from build123d import *

# Parameters (mm, degrees)
SKETCH2_R           = 10.9
SKETCH2_R_2         = 1.55
BOSS_EXTRUDE1_DEPTH = 4.5
SKETCH3_R           = 6.25
SKETCH3_R_2         = 2.1
BOSS_EXTRUDE2_DEPTH = 6.5
CUT_EXTRUDE2_START  = -9.5
SKETCH6_R           = 2.1
CUT_EXTRUDE2_DEPTH  = 9.5
SKETCH7_R           = 3.6
CUT_EXTRUDE3_DEPTH  = 2.9
CUT_EXTRUDE4_DEPTH  = 2.8
CHAMFER2_SIZE       = 0.5
SKETCH11_R          = 1.55
CUT_EXTRUDE5_DEPTH  = 5.5
SKETCH14_W          = 2.8
SKETCH14_H          = 6.2
CUT_EXTRUDE6_DEPTH  = 6.4
CUT_EXTRUDE8_DEPTH  = 6.2
CHAMFER3_SIZE       = 0.4
CHAMFER4_SIZE       = 0.4
SKETCH19_W          = 2.5
SKETCH19_H          = 7
BOSS_EXTRUDE4_DEPTH = 10
FILLET5_R           = 3
CUT_EXTRUDE9_DEPTH  = 6.5
CUT_EXTRUDE10_START = -87
SKETCH21_R          = 1.55
CUT_EXTRUDE10_DEPTH = 87


with BuildPart() as part:
    # Sketch2 → Boss-Extrude1 (new body)
    with BuildSketch(Plane.XY):
        Circle(SKETCH2_R)
        with Locations((0, 8)):
            Circle(SKETCH2_R_2, mode=Mode.SUBTRACT)
        with Locations((0, -8)):
            Circle(SKETCH2_R_2, mode=Mode.SUBTRACT)
    extrude(amount=BOSS_EXTRUDE1_DEPTH)

    # Sketch3 → Boss-Extrude2 (add)
    with BuildSketch(Plane(origin=(0, 0, 0), x_dir=(-1, 0, 0), z_dir=(0, 0, -1))):
        with Locations(Location((0, 0, 0), (0, 0, 180))):
            Circle(SKETCH3_R)
        with Locations(Location((0, 0, 0), (0, 0, 180))):
            Circle(SKETCH3_R_2, mode=Mode.SUBTRACT)
    extrude(amount=BOSS_EXTRUDE2_DEPTH)

    # Sketch6 → Cut-Extrude2 (cut)
    with BuildSketch(Plane(origin=(0, 0, 0), x_dir=(-1, 0, 0), z_dir=(0, 0, -1)).offset(CUT_EXTRUDE2_START)):
        with Locations(Location((0, 0, 0), (0, 0, 180))):
            Circle(SKETCH6_R)
    extrude(amount=CUT_EXTRUDE2_DEPTH, mode=Mode.SUBTRACT)

    # Sketch7 → Cut-Extrude3 (cut)
    with BuildSketch(Plane.XY.offset(4.5)):
        Circle(SKETCH7_R)
    extrude(amount=-CUT_EXTRUDE3_DEPTH, mode=Mode.SUBTRACT)

    # Sketch8 → Cut-Extrude4 (cut)
    with BuildSketch(Plane.XY.offset(4.5)):
        Polygon((1.58395502, 5.181415279), (3.232943481, 7.962452926), (1.64898846, 10.781037646), (-1.58395502, 10.818584721), (-3.232943481, 8.037547074), (-1.64898846, 5.218962354), align=None)
        Polygon((3.233098906, -8.020119499), (1.633973451, -5.210113964), (-1.599125456, -5.189994464), (-3.233098906, -7.979880501), (-1.633973451, -10.789886036), (1.599125456, -10.810005536), align=None)
    extrude(amount=-CUT_EXTRUDE4_DEPTH, mode=Mode.SUBTRACT)

    # Chamfer2
    chamfer2_edges = [part.edges().sort_by_distance(p)[0] for p in [
        (-3.6, 0, 4.5),
    ]]
    chamfer(chamfer2_edges, length=CHAMFER2_SIZE)

    # Sketch11 → Cut-Extrude5 (cut, symmetric)
    with BuildSketch(Plane(origin=(-6.25, 0, 0), x_dir=(0, 1, 0), z_dir=(-1, 0, 0))):
        with Locations(Location((0, 3.215789821, 0), (0, 0, 270))):
            Circle(SKETCH11_R)
    extrude(amount=CUT_EXTRUDE5_DEPTH, both=True, mode=Mode.SUBTRACT)

    # Sketch14 → Cut-Extrude6 (cut)
    with BuildSketch(Plane(origin=(0, 0, -6.5), x_dir=(-1, 0, 0), z_dir=(0, 0, -1))):
        with Locations((3.35, 0)):
            Rectangle(SKETCH14_W, SKETCH14_H)
    extrude(amount=-CUT_EXTRUDE6_DEPTH, mode=Mode.SUBTRACT)

    # Sketch17 → Cut-Extrude8 (cut)
    with BuildSketch(Plane.XY.offset(1.7)):
        Polygon((1.655062081, 10.777427379), (-1.577791627, 10.822039496), (-3.232853707, 8.044612117), (-1.655062081, 5.222572621), (1.577791627, 5.177960504), (3.232853707, 7.955387883), align=None)
    extrude(amount=CUT_EXTRUDE8_DEPTH, mode=Mode.SUBTRACT)

    # Chamfer3
    chamfer3_edges = [part.edges().sort_by_distance(p)[0] for p in [
        (3.231903858, 7.96069959, 4.5),
        (-1.649987082, 5.220739361, 4.5),
        (1.581916776, 5.181438951, 4.5),
        (-3.231903858, 8.03930041, 4.5),
        (-3.231858971, 8.042832931, 4.5),
        (0.771107805, 5.189092426, 4.5),
        (2.049929575, 10.07116703, 4.5),
        (1.578835079, 5.179711564, 4.5),
        (3.231858971, 7.957167069, 4.5),
        (-2.81987127, 8.737654839, 4.5),
        (-2.048763464, 5.926747264, 4.5),
        (-1.653023892, 5.222544495, 4.5),
        (2.81987127, 7.262345161, 4.5),
        (-10.899984913, 0.01813521, 4.5),
        (8.259417425, -7.112807026, 4.5),
        (2.837704165, 8.665765509, 4.5),
        (-2.006564209, 10.105849554, 4.5),
        (-2.837704165, 7.334234491, 4.5),
        (-0.842282238, 5.20959335, 4.5),
        (1.995421926, 5.87535886, 4.5),
        (-2.437601998, -9.377738754, 4.5),
        (2.42507938, -9.399751703, 4.5),
        (2.433536179, -6.615116731, 4.5),
        (0.017423997, -5.200054214, 4.5),
        (-2.416112181, -6.584937483, 4.5),
    ]]
    chamfer(chamfer3_edges, length=CHAMFER3_SIZE)

    # Chamfer4
    chamfer4_edges = [part.edges().sort_by_distance(p)[0] for p in [
        (-2.1, 0, 1.6),
    ]]
    chamfer(chamfer4_edges, length=CHAMFER4_SIZE)

    # Sketch19 → Boss-Extrude4 (add)
    with BuildSketch(Plane(origin=(0, 0, -6.5), x_dir=(-1, 0, 0), z_dir=(0, 0, -1))):
        with Locations((6.327927724, 0)):
            Rectangle(SKETCH19_W, SKETCH19_H)
    extrude(amount=-BOSS_EXTRUDE4_DEPTH)

    # Fillet5
    fillet5_edges = [part.edges().sort_by_distance(p)[0] for p in [
        (-5.178078794, -3.5, -3.25),
        (-5.178078794, 3.5, -3.25),
    ]]
    fillet(fillet5_edges, radius=FILLET5_R)

    # Sketch20 → Cut-Extrude9 (cut)
    with BuildSketch(Plane(origin=(0, 0, -6.5), x_dir=(-1, 0, 0), z_dir=(0, 0, -1))):
        Polygon((1.674315781, 10.9), (-1.674315781, 10.9), (-3.348631561, 8), (-1.674315781, 5.1), (1.674315781, 5.1), (3.348631561, 8), align=None)
        Polygon((1.674315781, -5.1), (-1.674315781, -5.1), (-3.348631561, -8), (-1.674315781, -10.9), (1.674315781, -10.9), (3.348631561, -8), align=None)
    extrude(amount=-CUT_EXTRUDE9_DEPTH, mode=Mode.SUBTRACT)

    # Sketch21 → Cut-Extrude10 (cut)
    with BuildSketch(Plane(origin=(-5.077927724, 0, 0), x_dir=(0, 0, -1), z_dir=(1, 0, 0)).offset(CUT_EXTRUDE10_START)):
        with Locations(Location((3.215789821, 0, 0), (0, 0, 180))):
            Circle(SKETCH21_R)
    extrude(amount=CUT_EXTRUDE10_DEPTH, mode=Mode.SUBTRACT)


solid = part.part
Can you work these out from the model? Positions are in its coordinate system, mm. A direction names the side the tool comes from. Give positions to 0.01 mm unless a question says otherwise; leave off trailing zeros. Write each loop counter-clockwise with the first axis right and the second up, starting at its lowest first coordinate (ties: lowest second). Pieces come first, ordered by that corner, then holes. Notation, with made-up numbers: (8, -30) -> (61, -30) arc R20 ccw to (61, -16) -> close; hole circle Ø3 at (-22, 85.5). An arc over 180 degrees is marked (long way). Answer as a JSON object with one key per item and string values. Group by question number.
Item 1: For faces 4 (the face through (-7.578, -2, -3)), 5 (the face through (-2, 10.12, 2.92)), 6 (the face through (-5.44, 3.726, -3.204)), which set-ups out of +Z, -Z, +X, -X, +Y, -Y let a thin tool reach every point of the face, with its end or its side?
Item 2: Suppose I cut it at A-A (z = 2). State how many separate pieces and enclosed holes the cut face has, plus the area to 3 significant figures.
Item 3: Please list where these lines run through material, in increasing order: line 1 (X direction, y = 1.5, z = -2); line 2 (Z direction, x = -8.5, y = -1.25); line 3 (Y direction, x = -2, z = -3.75). Write a range as [from, to].
Item 4: We'd pull the mould along X, two halves only. Please class faces 1 (the face through (5.03, -9.67, 1.72)), 2 (the face through (-10.61, 0.23, 4.39)), 3 (the face through (3.06, 8.673, 4.297)): +X half, -X half, draft (parallel to the pull), parting line (faces both ways), or undercut.
Item 5: Suppose I cut it at C-C (z = 0.5). Please give me the cut outline in (x, y), plus the area to 3 significant figures.
Item 6: Suppose I cut it at B-B (y = 0). Please give me the cut outline in (x, z), plus the area to 3 significant figures.
Item 7: I'm going to push flat-ended pins straight in: P1, Ø4, axis at x = 0, y = 0, coming from the +Z side; P2, Ø1.4, axis at x = -3, z = -3, coming from the +Y side; P3, Ø11.5, axis at x = 0, y = 0, coming from the +Z side; P4, Ø3, axis at x = -3, z = -3.5, coming from the -Y side. Where does each tip first touch, or does it pass through?
Findings:
{
 "1": {"face 4": "-Z, -X, +Y, -Y", "face 5": "+Z", "face 6": "-Z, -X, +Y"},
 "2": {"separate pieces": "3", "enclosed holes": "1", "area": "278 mm²"},
 "3": {"line 1": "x = [-7.58, -4.75], [-1.95, -1.47], [1.47, 6.07]", "line 2": "z = [0, 4.5]", "line 3": "y = [-5.66, -3.1], [3.1, 5.66]"},
 "4": {"face 1": "parting line", "face 2": "-X half", "face 3": "undercut"},
 "5": {"outline": "circle Ø21.8 at (0, 0); hole circle Ø4.2 at (0, 0); hole circle Ø3.1 at (0, -8); hole circle Ø3.1 at (0, 8)", "area": "344 mm²"},
 "6": {"outline": "(-10.9, 0) -> (-7.58, 0) -> (-7.58, -1.67) -> (-4.75, -1.67) -> (-4.75, -0.1) -> (-2.1, -0.1) -> (-2.1, 1.2) -> (-2.5, 1.6) -> (-3.6, 1.6) -> (-3.6, 4) -> (-4.1, 4.5) -> (-10.5, 4.5) -> (-10.9, 4.1) -> close; (-7.58, -6.5) -> (-4.75, -6.5) -> (-4.75, -4.77) -> (-7.58, -4.77) -> close; (2.1, -6.5) -> (6.25, -6.5) -> (6.25, 0) -> (10.9, 0) -> (10.9, 4.1) -> (10.5, 4.5) -> (4.1, 4.5) -> (3.6, 4) -> (3.6, 1.6) -> (2.5, 1.6) -> (2.1, 1.2) -> close", "area": "107 mm²"},
 "7": {"P1": "passes through", "P2": "stops at y = 5.81", "P3": "stops at z = 4.5", "P4": "stops at y = -5.88"}
}
